Autodesk Inventor part; units mm, degrees
ref_plane "YZ Plane" through (0, 0, 0) normal (1, 0, 0) x (0, 1, 0)
ref_plane "XZ Plane" through (0, 0, 0) normal (0, 1, 0) x (-1, 0, 0)
ref_plane "XY Plane" through (0, 0, 0) normal (0, 0, 1) x (1, 0, 0)
sketch "Sketch1" plane through (0, 0, 0) normal (0, 0, 1) x (1, 0, 0)
  line L0 (0, 0) -> (-30, 0)
  line L1 (-30, 40) -> (0, 40)
  line L2 (-36.1318, 34) -> (13.8682, 34) construction
  arc A0 (0, 30) -> (0, 38) centre (0, 34) ccw
  circle A1 centre (-30, 34) radius 4 construction
  line L3 (-30, 30) -> (0, 30) construction
  line L4 (-30, 38) -> (-26, 34)
  line L5 (-30, 30) -> (-26, 34)
  line L6 (0, 40) -> (0, 38)
  line L7 (0, 30) -> (0, 0)
  line L8 (-30, 0) -> (-30, 30)
  line L9 (-30, 38) -> (-30, 40)
  dimension "d0" = 30
  dimension "d1" = 40
  dimension "d3" = 6
  dimension "d4" = 8
  dimension "d5" = 8
  dimension "d6" = 30
extrude "Extrusion1" add sketch "Sketch1" along normal blind 3
sketch "Sketch3" plane through (0, 0, 3) normal (0, 0, 1) x (1, 0, 0)
  line L0 (-30, 40) -> (0, 40) construction
  line L1 (-30, 0) -> (-30, 30) construction
  line L2 (0, 0) -> (-30, 0) construction
  line L3 (-15.0586, 25.9999) -> (-30, 25.9849) construction
  line L4 (-28.1581, 25.9868) -> (-7.691, 25.9868)
  line L5 (-7.691, 25.9868) -> (-7.691, 23.9868)
  line L6 (-28.1581, 23.9868) -> (-28.1581, 25.9868)
  line L7 (-7.691, 24.9868) -> (-1.5179, 24.9868) construction
  line L8 (-7.691, 25.9868) -> (-7.691, 27.4868)
  line L9 (-7.691, 27.4868) -> (-3.3609, 24.9868)
  line L10 (-7.691, 23.9868) -> (-7.691, 22.4868)
  line L11 (-7.691, 22.4868) -> (-3.3609, 24.9868)
  line L12 (-14.0467, 18.4868) -> (-16.0467, 18.4868)
  line L13 (-16.0467, 18.4868) -> (-16.0467, 22.9868)
  line L14 (-16.0467, 22.9868) -> (-14.0467, 22.9868)
  line L15 (-14.0467, 22.9868) -> (-14.0467, 18.4868)
  line L16 (-14.0467, 18.4868) -> (-16.0467, 22.9868) construction
  line L17 (-16.0467, 18.4868) -> (-14.0467, 22.9868) construction
  line L18 (-15, 0) -> (-15.0135, 6) construction
  line L19 (-15.0135, 6) -> (-28.7905, 6) construction
  line L20 (-13.75, 6.5) -> (-18.25, 6.5)
  line L21 (-18.25, 6.5) -> (-18.25, 4.5)
  line L22 (-18.25, 4.5) -> (-13.75, 4.5)
  line L23 (-13.75, 4.5) -> (-13.75, 6.5)
  line L24 (-19.75, 6.5) -> (-24.25, 6.5)
  line L25 (-19.75, 4.5) -> (-19.75, 6.5)
  line L26 (-24.25, 4.5) -> (-19.75, 4.5)
  line L27 (-24.25, 6.5) -> (-24.25, 4.5)
  line L28 (-24.25, 5.5) -> (-29.2128, 5.5) construction
  line L29 (-24.25, 6.5) -> (-24.25, 8)
  line L30 (-24.25, 8) -> (-28.5801, 5.5)
  line L31 (-24.25, 4.5) -> (-24.25, 3)
  line L32 (-24.25, 3) -> (-28.5801, 5.5)
  line L33 (-16.616, 36.5) -> (-11.3751, 36.5) construction
  line L34 (-11.3751, 36.5) -> (-11.3751, 28.9531) construction
  line L35 (-11.3751, 28.9531) -> (-16.616, 28.9531) construction
  line L36 (-16.616, 28.9531) -> (-16.616, 36.5) construction
  line L37 (-16.25, 40) -> (-16.25, 36.4806) construction
  line L38 (-28.1581, 23.9868) -> (-7.691, 23.9868)
  line L39 (-16.0467, 17.4868) -> (-14.0467, 17.4868)
  line L40 (-14.0467, 17.4868) -> (-14.0467, 12.9868)
  line L41 (-16.0467, 12.9868) -> (-16.0467, 17.4868)
  line L42 (-14.0467, 12.9868) -> (-16.0467, 12.9868)
  line L43 (-16.0467, 12.9868) -> (-14.0467, 17.4868) construction
  line L44 (-14.0467, 12.9868) -> (-16.0467, 17.4868) construction
  line L45 (-16.0467, 11.9868) -> (-14.0467, 11.9868)
  line L46 (-14.0467, 11.9868) -> (-14.0467, 7.4868)
  line L47 (-16.0467, 7.4868) -> (-16.0467, 11.9868)
  line L48 (-14.0467, 7.4868) -> (-16.0467, 7.4868)
  line L49 (-16.0467, 7.4868) -> (-14.0467, 11.9868) construction
  line L50 (-14.0467, 7.4868) -> (-16.0467, 11.9868) construction
  line L51 (-13.8725, 30.4) -> (-16.2354, 30.4)
  line L52 (-16.2354, 30.4) -> (-16.2354, 31.0229)
  line L53 (-16.2354, 31.0229) -> (-15.4593, 31.0229)
  line L54 (-15.4593, 31.0229) -> (-15.4593, 35.8771)
  line L55 (-15.4593, 35.8771) -> (-16.2354, 35.8771)
  line L56 (-16.2354, 35.8771) -> (-16.2354, 36.5)
  line L57 (-16.2354, 36.5) -> (-13.8725, 36.5)
  line L58 (-13.8725, 36.5) -> (-13.8725, 35.8771)
  line L59 (-13.8725, 35.8771) -> (-14.6486, 35.8771)
  line L60 (-14.6486, 35.8771) -> (-14.6486, 31.0229)
  line L61 (-14.6486, 31.0229) -> (-13.8725, 31.0229)
  line L62 (-13.8725, 31.0229) -> (-13.8725, 30.4)
  point P0 (-15.0467, 20.7368)
  point P1 (-15.0467, 15.2368)
  point P2 (-15.0467, 9.7368)
  point P3 (-15, 40)
  point P4 (-15, 40)
  dimension "d10" = 26
  dimension "d11" = 2
  dimension "d12" = 1.5
  dimension "d13" = 5
  dimension "d14" = 1.5
  dimension "d15" = 2
  dimension "d16" = 4.5
  dimension "d24" = 6
  dimension "d25" = 4.5
  dimension "d26" = 2
  dimension "d29" = 6
  dimension "d34" = 1.5
  dimension "d35" = 5
  dimension "d36" = 1.5
  dimension "d39" = 8
  dimension "d40" = 1
  dimension "d48" = 5.5
  dimension "d53" = 3.5
  dimension "d54" = 14
extrude "Extrusion2" cut sketch "Sketch3" against normal blind 1
properties part number "MS_I[203] text"
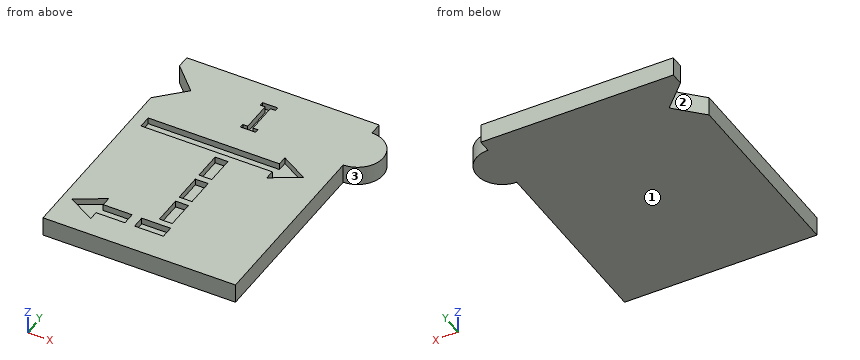
Work out the finished part from the listing and answer in its coordinate system (mm). Face numbers are marked on the shaded views. Round coordinates to 2 decimals unless told otherwise and drop trailing zeros. Write each loop counter-clockwise with the first axis right and the second up, starting at its lowest first coordinate (ties: lowest second). Pieces come first, ordered by that corner, then holes.
1) A cutting plane is placed at A-A (z = 0.45). Give the vertices of the cut face in (x, y), plus the area to 3 significant figures.
2) Straight lines are drawn through the part: line 1 (Y direction, x = -23, z = 2.3); line 2 (X direction, y = 21, z = 2.4); line 3 (Z direction, x = -16, y = 30.5). For each, find the intervals that lie inside material, in ascending order.
3) A cutting plane is placed at C-C (x = -17). Give the vertices of the cut face in (y, z), plus the area to 3 significant figures.
4) A cutting plane is placed at B-B (y = 20). Give the vertices of the cut face in (x, z).
5) The mould has two halves that part along Y. Classify the marked faces 1, 2 and 3: pulls with the +Y half, pulls with the -Y half, needs draft (parallel to the pull), parting line crosses it, or undercut.
6) Given pin 1 Ø1.1 at (y, z) = (34.5, 2.5) entering from -X; pin 2 Ø0.5 at (y, z) = (14.5, 2.5) entering from +X, each flat-ended and moving along its own axis, determine where each tip first touches the part or whether it passes through.
7) A cutting plane is placed at D-D (y = 35). Give the vertices of the cut face in (x, z), plus the area to 3 significant figures.
Completed:
1. outline: (-30, 0) - (0, 0) - (0, 30) arc R4 ccw to (0, 38) - (0, 40) - (-30, 40) - (-30, 38) - (-26, 34) - (-30, 30) - close
1. area: 1,210 mm2
2. line 1: y = 0 to 4.5, 6.5 to 23.99, 25.99 to 40
2. line 2: x = -30 to -16.05, -14.05 to 0
2. line 3: z = 0 to 2
3. outline: (0, 0) - (40, 0) - (40, 3) - (25.99, 3) - (25.99, 2) - (23.99, 2) - (23.99, 3) - (6.5, 3) - (6.5, 2) - (4.5, 2) - (4.5, 3) - (0, 3) - close
3. area: 116 mm2
4. outline: (-30, 0) - (0, 0) - (0, 3) - (-14.05, 3) - (-14.05, 2) - (-16.05, 2) - (-16.05, 3) - (-30, 3) - close
5. face 1: needs draft
5. face 2: undercut
5. face 3: parting line crosses it
6. pin 1: stops at x = -27.05
6. pin 2: stops at x = 0
7. outline: (-27, 0) - (3.87, 0) - (3.87, 3) - (-14.65, 3) - (-14.65, 2) - (-15.46, 2) - (-15.46, 3) - (-27, 3) - close
7. area: 91.8 mm2
